Read the model definition and answer for the solid it produces. Units are mm, in the model's axes. Face numbers are marked on the shaded views. A direction names the side the tool comes from. Coordinates: 2 decimals unless noted, no trailing zeros. Write each loop counter-clockwise with the first axis right and the second up, starting at its lowest first coordinate (ties: lowest second). Pieces come first, ordered by that corner, then holes. Notation, with made-up numbers: (50.5, 70.5) -> (71.5, 70.5) arc R27 cw to (71.5, 107.5) -> close; hole circle Ø9 at (28, -10.5). An arc over 180 degrees is marked (long way). Use CSV: the item, a comma, the result in double quotes. Start each with the question number.
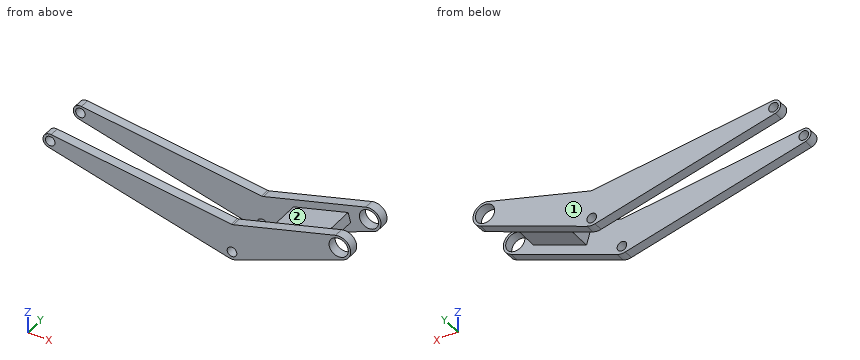
from build123d import *

# Parameters (mm, degrees)
BOSS_EXTRUDE3_DEPTH = 60
SKETCH4_R           = 10
SKETCH4_R_2         = 5
CUT_EXTRUDE2_DEPTH  = 98.5
SKETCH5_W           = 377.10594696
SKETCH5_H           = 125.451579965
CUT_EXTRUDE3_DEPTH  = 20
SKETCH6_R           = 5
CUT_EXTRUDE4_DEPTH  = 40.5


with BuildPart() as part:
    # Sketch1 → Boss-Extrude3 (new body)
    with BuildSketch(Plane(origin=(0, 0, 0), x_dir=(1, 0, 0), z_dir=(0, 1, 0))):
        with BuildLine():
            Line((-63.667210577, 7.268578883), (123.791080386, 54.947452974))
            ThreePointArc((123.791080386, 54.947452974), (128.085809082, 55.353988191), (132.30042121, 54.43365669))
            Line((132.30042121, 54.43365669), (242.697935991, 11.655551457))
            ThreePointArc((242.697935991, 11.655551457), (250.046544834, -3.933307136), (234.840986043, -12.045368899))
            Line((234.840986043, -12.045368899), (128.578230905, 17.424304308))
            ThreePointArc((128.578230905, 17.424304308), (127.586579666, 17.594270625), (126.58097714, 17.562266071))
            Line((126.58097714, 17.562266071), (-60.826924457, -7.434163985))
            ThreePointArc((-60.826924457, -7.434163985), (-69.182345376, -1.422554364), (-63.667210577, 7.268578883))
        make_face()
    extrude(amount=BOSS_EXTRUDE3_DEPTH)

    # Sketch4 → Cut-Extrude2 (cut, symmetric)
    with BuildSketch(Plane(origin=(0, 30, 0), x_dir=(1, 0, 0), z_dir=(0, 1, 0))):
        with Locations(Location((238.181508173, 0, 0), (0, 0, 270))):
            Circle(SKETCH4_R)
        with Locations(Location((-61.818491827, 0, 0), (0, 0, 270))):
            Circle(SKETCH4_R_2)
    extrude(amount=CUT_EXTRUDE2_DEPTH, both=True, mode=Mode.SUBTRACT)

    # Sketch5 → Cut-Extrude3 (cut, symmetric)
    with BuildSketch(Plane(origin=(0, 30, 0), x_dir=(1, 0, 0), z_dir=(0, 1, 0))):
        with Locations((90.046698809, 24.704131579)):
            Rectangle(SKETCH5_W, SKETCH5_H)
        Polygon((159.740207612, 16.633427142), (216.469846148, 0.900690808), (219.199055149, 10.741765928), (164.034407851, 32.117601172), align=None, mode=Mode.SUBTRACT)
    extrude(amount=CUT_EXTRUDE3_DEPTH, both=True, mode=Mode.SUBTRACT)

    # Sketch6 → Cut-Extrude4 (cut, symmetric)
    with BuildSketch(Plane(origin=(0, 30, 0), x_dir=(1, 0, 0), z_dir=(0, 1, 0))):
        with Locations(Location((127.242022054, 47.44112623, 0), (0, 0, 270))):
            Circle(SKETCH6_R)
    extrude(amount=CUT_EXTRUDE4_DEPTH, both=True, mode=Mode.SUBTRACT)


solid = part.part
1) Which of the six approach directions +Z, -Z, +X, -X, +Y, -Y give full straight-line access (tool end or side, diameter ignored) to the marked faces 1 and 2?
2) Each of these flat-tipped pins is pushed along its axis until it touches: pin 1 (13 mm diameter, centred on x = -61.82, z = 0, fed in from +Y); pin 2 (4 mm diameter, centred on y = 39, z = -11, fed in from +X); pin 3 (2 mm diameter, centred on x = 192, y = 34.5, fed in from +Z); pin 4 (8 mm diameter, centred on x = 127.24, z = -47.44, fed in from +Y). Where does it stop, or does it pass through?
3) Section B-B, the plane y = 32.5 is taken. Give the vertices of the cut face in (x, z), plus the area to 3 significant figures.
4) Section A-A, the plane x = 17 is taken. Give the vertices of the cut face in (y, z), plus the area to 3 significant figures.
5) Find the intervals of material crossed by line 1 along Y through (x, z) = (-43.5, -10); line 2 along Z through (x, y) = (78.5, 3.5); line 3 along Z through (x, y) = (190, 37), in increasing order.
6) Section C-C, the plane y = 53 is taken. Give the vertices of the cut face in (x, z).
7) Section D-D, the plane x = 102.5 is taken. Give the vertices of the cut face in (y, z).
The answers:
1,face 1,"+Z, -Z, +X, -X, +Y"
1,face 2,"+Z, -X"
2,pin 1,"stops at y = 60"
2,pin 2,"stops at x = 219.2"
2,pin 3,"stops at z = -7.41"
2,pin 4,"passes through"
3,outline,"(159.74, -16.63) -> (164.03, -32.12) -> (219.2, -10.74) -> (216.47, -0.9) -> close"
3,area,"774 mm^2"
4,outline,"(0, -27.79) -> (10, -27.79) -> (10, -2.95) -> (0, -2.95) -> close; (50, -27.79) -> (60, -27.79) -> (60, -2.95) -> (50, -2.95) -> close"
4,area,"497 mm^2"
5,line 1,"y = 0 to 10, 50 to 60"
5,line 2,"z = -43.43 to -11.15"
5,line 3,"z = -22.06 to -8.24"
6,outline,"(-63.67, -7.27) -> (123.79, -54.95) arc R14 ccw to (132.3, -54.43) -> (242.7, -11.66) arc R12.5 ccw to (234.84, 12.05) -> (128.58, -17.42) arc R5 cw to (126.58, -17.56) -> (-60.83, 7.43) arc R7.5 ccw to start; hole circle Ø10 at (-61.82, 0); hole circle Ø10 at (127.24, -47.44); hole circle Ø20 at (238.18, 0)"
7,outline,"(0, -49.53) -> (10, -49.53) -> (10, -14.35) -> (0, -14.35) -> close; (50, -49.53) -> (60, -49.53) -> (60, -14.35) -> (50, -14.35) -> close"
